Check sheet for the modelled part. Datum: model origin and axes. Units: mm. Face numbers are marked on the shaded views. A direction names the side the tool comes from. Give positions to 0.01 mm unless a question says otherwise; leave off trailing zeros. Loops run counter-clockwise (first coordinate to the right, second up) from the corner with the lowest first, then second, coordinate; pieces in that order, holes last. Notation, with made-up numbers: (-8, -38) - (27, -38) arc R11 ccw to (27, -22) - close; hole circle Ø9 at (4, -18.75). An arc over 180 degrees is marked (long way). Answer in a Markdown table with one row per item. Add a question column.
(1) Thickness scan on L1, parallel to Y at x = 0, z = 42; L2, parallel to Y at x = 0, z = 23; L3, parallel to Z at x = 14, y = -32.5. Record the ranges inside material, lowest first.
(2) Sectioned sample at A-A on z = 48. Enter the section's corners in (x, y).
(3) Go/stop test with flat-tipped pins: P1, Ø8, axis at x = 25.5, z = 35.5, coming from the +Y side; P2, Ø4.5, axis at x = -4, z = 50, coming from the -Y side; P3, Ø4, axis at y = 33.5, z = 39, coming from the -X side. Record where each tip stops, or that it passes through.
(4) Set-up check for the marked faces 4, 5 and 6: record each of +Z, -Z, +X, -X, +Y, -Y from which the full face is reachable in a straight line by a thin tool's end or side.
(5) Draft check along Y on the marked faces 1, 2 and 3. Enter one of: released by +Y, released by -Y, zero draft, split by the parting line, or undercut.
(6) Sectioned sample at D-D on x = -8.5. Enter the section's corners in (y, z), then the cut area to 3 significant figures.
(7) Sectioned sample at C-C on z = 6.5. Enter the section's corners in (x, y).
(8) Sectioned sample at B-B on y = 0. Enter the section's corners in (x, z), then the cut area to 3 significant figures.
from build123d import *

# Parameters (mm, degrees)
F1_DEPTH = 40
F2_W     = 30
F2_H     = 30
F3_DEPTH = 15
F4_R     = 10
F5_DEPTH = 40


with BuildPart() as f1:
    # F0 (on Top) → F1 (new body)
    with BuildSketch(Plane.XY):
        Polygon((38.971143, -22.5), (38.971143, 22.5), (0, 45), (-38.971143, 22.5), (-38.971143, -22.5), (0, -45), align=None)
    extrude(amount=F1_DEPTH)

    # F2 (on face) → F3 (join)
    with BuildSketch(Plane.XY.offset(40)):
        Rectangle(F2_W, F2_H)
    extrude(amount=F3_DEPTH)

    # F4 (on face) → F5 (cut)
    with BuildSketch(Plane.XY.offset(55)):
        Circle(F4_R)
    extrude(amount=-F5_DEPTH, mode=Mode.SUBTRACT)


solid = f1.part
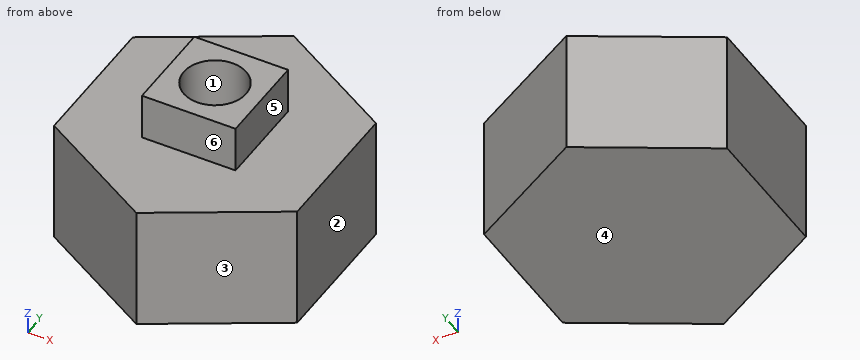
Reply:
| question | item | result |
|---|---|---|
| 1 | L1 | -15 to -10, 10 to 15 |
| 1 | L2 | -45 to -10, 10 to 45 |
| 1 | L3 | 0 to 40 |
| 2 | outline | (-15, -15) - (15, -15) - (15, 15) - (-15, 15) - close; hole circle Ø20 at (0, 0) |
| 3 | P1 | y = 32.59 |
| 3 | P2 | y = -15 |
| 3 | P3 | x = -23.38 |
| 4 | face 4 | -Z, +X, -X, +Y, -Y |
| 4 | face 5 | +Z, +X, +Y, -Y |
| 4 | face 6 | +Z, +X, -X, -Y |
| 5 | face 1 | undercut |
| 5 | face 2 | zero draft |
| 5 | face 3 | released by -Y |
| 6 | outline | (-40.09, 0) - (40.09, 0) - (40.09, 40) - (15, 40) - (15, 55) - (5.27, 55) - (5.27, 15) - (-5.27, 15) - (-5.27, 55) - (-15, 55) - (-15, 40) - (-40.09, 40) - close |
| 6 | area | 3,240 mm^2 |
| 7 | outline | (-38.97, -22.5) - (0, -45) - (38.97, -22.5) - (38.97, 22.5) - (0, 45) - (-38.97, 22.5) - close |
| 8 | outline | (-38.97, 0) - (38.97, 0) - (38.97, 40) - (15, 40) - (15, 55) - (10, 55) - (10, 15) - (-10, 15) - (-10, 55) - (-15, 55) - (-15, 40) - (-38.97, 40) - close |
| 8 | area | 2,770 mm^2 |
